Read the model definition and answer for the solid it produces. Units are mm, in the model's axes. A direction names the side the tool comes from. Coordinates: 2 decimals unless noted, no trailing zeros. Write each loop counter-clockwise with the first axis right and the second up, starting at its lowest first coordinate (ties: lowest second). Pieces come first, ordered by that corner, then holes.
(1) The part is cut by section A-A, the plane z = -70.5. Determine the outline of the cut face in (x, y), and give its area (3 significant figures).
(2) Determine the mould class of faces 1 (the cylindrical face through (-0.867, -3.905, 1.225)), 2 (the conical face through (-0.034, 0.261, -75.167)), 3 (the flat face through (2, 0, -87.5)) for opening direction Y: pulls with the +Y half, pulls with the -Y half, needs draft (parallel to the pull), parting line crosses it, or undercut.
(3) Straight lines are drawn through the part: line 1 along Y through (x, z) = (0, 79.5); line 2 along X through (y, z) = (-0.5, 64.5); line 3 along Z through (x, y) = (-0.5, 0). For each, find the intervals that lie inside material, in ascending order.
(4) Which of the six approach directions +Z, -Z, +X, -X, +Y, -Y give full straight-line access (tool end or side, diameter ignored) to faces 4 (the cylindrical face through (-1.216, 1.115, -81.67)), 5 (the flat face through (2, 0, 87.5)), 6 (the cylindrical face through (-1.216, 1.115, 81.83))?
```python
from build123d import *

# Parameters (mm, degrees)
SKETCH_1_R      = 4
SKETCH_1_R_2    = 2
EXTRUDE_1_DEPTH = 87.5


# Read off the part's stored shape, not the designer's step: M4x0.7 ねじ穴1
with BuildPart() as part:
    # ｽｹｯﾁ1 → ﾎﾞｽ - 押し出し1 (new, symmetric)
    # profile 1 of 2: a face of its own
    with BuildSketch(Plane.XY):
        Circle(SKETCH_1_R)
        Circle(SKETCH_1_R_2, mode=Mode.SUBTRACT)
    # profile 2 of 2: a face of its own
    with BuildSketch(Plane.XY):
        Circle(SKETCH_1_R_2)
    extrude(amount=EXTRUDE_1_DEPTH, both=True)

    # M4x0.7 ねじ穴1 outline → M4x0.7 ねじ穴1 (revolve, cut)
    with BuildSketch(Plane.XZ):
        Polygon((1.65, -76), (0, -75.008579979), (0, -87.5), (1.65, -87.5), align=None)
        Polygon((0, 87.5), (0, 75.008579979), (1.65, 76), (1.65, 87.5), align=None)
    revolve(axis=Axis((0, 0, 0), (0, 0, 1)), mode=Mode.SUBTRACT)


solid = part.part
```
Computed:
1. outline: circle Ø8 at (0, 0)
1. area: 50.3 mm2
2. face 1: parting line crosses it
2. face 2: undercut
2. face 3: needs draft
3. line 1: y = -4 to -1.65, 1.65 to 4
3. line 2: x = -3.97 to 3.97
3. line 3: z = -75.31 to 75.31
4. face 4: -Z
4. face 5: +Z, +X, -X, +Y, -Y
4. face 6: +Z
